Part model, mm, in its own coordinate system. Face numbers are marked on the shaded views. A direction names the side the tool comes from. Give positions to 0.01 mm unless a question says otherwise; leave off trailing zeros. Order: outer loops, then holes, each group sorted by start corner. A loop starts at its lowest first (then second) coordinate and runs counter-clockwise, first axis right, second up. Notation, with made-up numbers: (34, 88.25) - (71, 88.25) arc R17 cw to (71, 118.25) - close; hole circle Ø4 at (18, -35). An arc over 180 degrees is marked (long way). One line per item, written item: value.
```python
from build123d import *

# Parameters (mm, degrees)
BOSS_EXTRUDE1_DEPTH      = 55
BOSS_EXTRUDE2_START      = 13
BOSS_EXTRUDE2_DEPTH      = 13
BOSS_EXTRUDE3_REACH      = 93.1
BOSS_EXTRUDE3_END_RADIUS = 40
SKETCH3_R                = 8
HOLE1_D                  = 9


with BuildPart() as part:
    # Sketch1 → Boss-Extrude1 (new, symmetric)
    with BuildSketch(Plane.XY):
        with BuildLine():
            Line((5, 39.686269666), (5, 29.580398915))
            ThreePointArc((5, 29.580398915), (30, 0), (5, -29.580398915))
            Line((5, -29.580398915), (5, -39.686269666))
            ThreePointArc((5, -39.686269666), (40, 0), (5, 39.686269666))
        make_face()
    extrude(amount=BOSS_EXTRUDE1_DEPTH, both=True)

    # Sketch2 → Boss-Extrude2 (add)
    with BuildSketch(Plane.XY.offset(55).offset(BOSS_EXTRUDE2_START)):
        with BuildLine():
            Line((5, 29.580398915), (5, 47.236109069))
            ThreePointArc((5, 47.236109069), (47.5, 0), (5, -47.236109069))
            Line((5, -47.236109069), (5, -29.580398915))
            ThreePointArc((5, -29.580398915), (30, 0), (5, 29.580398915))
        make_face()
    boss_extrude2 = extrude(amount=-BOSS_EXTRUDE2_DEPTH)

    # Mirror1: Boss-Extrude2 across plane
    add(boss_extrude2.mirror(Plane.XY))

    # Boss-Extrude3: up to this cylinder (the profile starts outside it)
    boss_extrude3_end = Plane(origin=(0, 0, 0), z_dir=(0, 0, -1)) * Cylinder(BOSS_EXTRUDE3_END_RADIUS, 267.2, mode=Mode.PRIVATE)
    # Sketch3 → Boss-Extrude3 (add, up to the surface)
    with BuildSketch(Plane(origin=(43, 0, 0), x_dir=(0, 0, -1), z_dir=(1, 0, 0)), mode=Mode.PRIVATE) as boss_extrude3_sk1:
        Circle(SKETCH3_R)
    boss_extrude3_tool1 = extrude(boss_extrude3_sk1.sketch, amount=-BOSS_EXTRUDE3_REACH, mode=Mode.PRIVATE) - boss_extrude3_end
    add(boss_extrude3_tool1.solids().sort_by_distance((43, 0, 0))[0])

    # Hole1 (through all)
    with Locations(Plane(origin=(43, 0, 0), x_dir=(0, 0, -1), z_dir=(1, 0, 0))):
        with Locations((0, 0)):
            Hole(HOLE1_D / 2)


solid = part.part
```
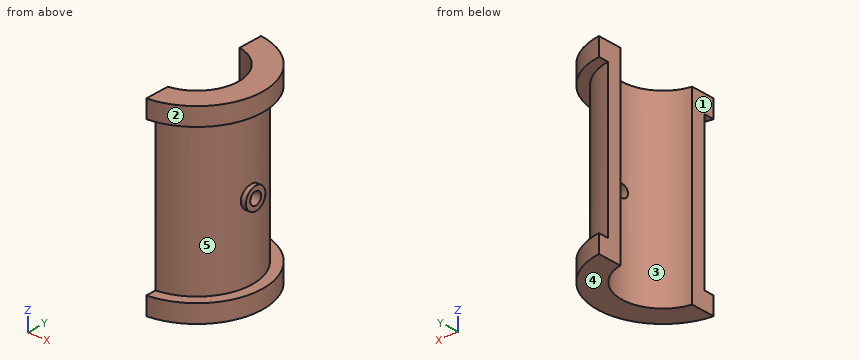
1) Cut at D-D, the plane y = 17. Give the cut face in (x, z).
Outcome:
outline: (24.72, -68) - (44.35, -68) - (44.35, -55) - (36.21, -55) - (36.21, 55) - (44.35, 55) - (44.35, 68) - (24.72, 68) - close
2) Mould opens along Y. For the marked faces 1, 2 and 3 say: released by +Y, released by -Y, zero draft, split by the parting line, or undercut.
Outcome:
face 1: zero draft
face 2: split by the parting line
face 3: undercut
3) Cut at B-B, the plane y = 0. Give the cut face in (x, z), then the cut area to 3 significant figures.
Outcome:
outline: (30, -68) - (47.5, -68) - (47.5, -55) - (40, -55) - (40, -8) - (43, -8) - (43, -4.5) - (30, -4.5) - close; (30, 4.5) - (43, 4.5) - (43, 8) - (40, 8) - (40, 55) - (47.5, 55) - (47.5, 68) - (30, 68) - close
area: 1,490 mm^2
4) Drill centre lines: line 1 along Z through (x, y) = (39, 0); line 2 along Y through (x, z) = (24.5, -60); line 3 along Y through (x, z) = (11, -32). Where is each one in solid material? Low to high. Write a range as from..to.
Outcome:
line 1: z = -68..-4.5, 4.5..68
line 2: y = -40.69..-17.31, 17.31..40.69
line 3: y = -38.46..-27.91, 27.91..38.46
5) Cut at C-C, the plane x = 19. Give the cut face in (y, z), then the cut area to 3 significant figures.
Outcome:
outline: (-43.53, -68) - (-23.22, -68) - (-23.22, 68) - (-43.53, 68) - (-43.53, 55) - (-35.2, 55) - (-35.2, -55) - (-43.53, -55) - close; (23.22, -68) - (43.53, -68) - (43.53, -55) - (35.2, -55) - (35.2, 55) - (43.53, 55) - (43.53, 68) - (23.22, 68) - close
area: 3,690 mm^2
6) Which spindle directions (+Z, -Z, +X, -X, +Y, -Y) get a long thin tool onto all of the face, cutting with end or side? Do the marked faces 4 and 5. Say none if no direction does.
Outcome:
face 4: -Z, +X, -X, +Y, -Y
face 5: +X
7) Pin check, flat tips, straight feed: pin 1 (4 mm diameter, centred on x = 24, y = -15.5, fed in from -Z); pin 2 (2 mm diameter, centred on x = 20.5, z = 16.5, fed in from +Y); pin 3 (13 mm diameter, centred on y = 4, z = -1.5, fed in from +X); pin 4 (8 mm diameter, centred on y = 0, z = 0, fed in from +X). Stop position of each tip, or through.
Outcome:
pin 1: stops at z = -68
pin 2: stops at y = 34.92
pin 3: stops at x = 43
pin 4: passes through
8) Cut at A-A, the plane z = 0. Give the cut face in (x, y), then the cut area to 3 significant figures.
Outcome:
outline: (5, -39.69) arc R40 ccw to (39.19, -8) - (43, -8) - (43, -4.5) - (29.66, -4.5) arc R30 cw to (5, -29.58) - close; (5, 29.58) arc R30 cw to (29.66, 4.5) - (43, 4.5) - (43, 8) - (39.19, 8) arc R40 ccw to (5, 39.69) - close
area: 933 mm^2
